from build123d import *

# Parameters (mm, degrees)
F0_W     = 67.3
F0_H     = 105.5
F1_DEPTH = 3
F2_W     = 56.2
F2_H     = 97.6
F3_DEPTH = 0.3
F4_W     = 48.5
F4_H     = 3
F5_DEPTH = 2


with BuildPart() as f1:
    # F0 (on Top) → F1 (new body)
    with BuildSketch(Plane.XY):
        with Locations((11.620628, 4.456163)):
            Rectangle(F0_W, F0_H)
    extrude(amount=F1_DEPTH)

    # F2 (on face) → F3 (cut)
    with BuildSketch(Plane.XY.offset(3)):
        with Locations((13.620628, 4.306163)):
            Rectangle(F2_W, F2_H)
    extrude(amount=-F3_DEPTH, mode=Mode.SUBTRACT)

    # F4 (on face) → F5 (join)
    with BuildSketch(Plane(origin=(-22.029372, 0, 0), x_dir=(0, -1, 0), z_dir=(-1, 0, 0))):
        with Locations((-14.056163, 1.5)):
            Rectangle(F4_W, F4_H)
    extrude(amount=F5_DEPTH)


solid = f1.part
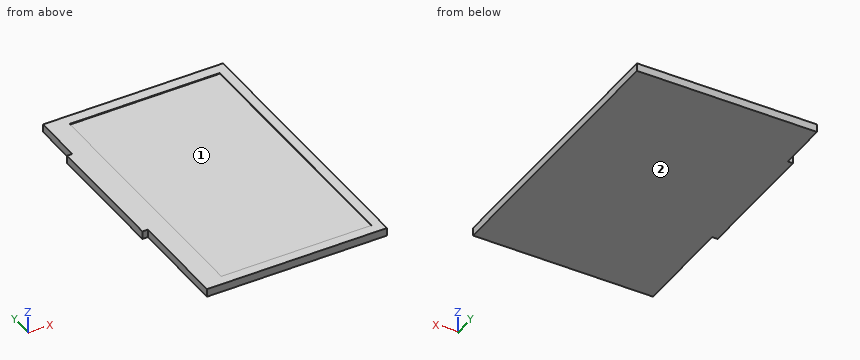
Verification items for the finished model (mm, model axes). Face numbers are marked on the shaded views. Coordinates: 2 decimals unless noted, no trailing zeros. Order: outer loops, then holes, each group sorted by start corner. A loop starts at its lowest first (then second) coordinate and runs counter-clockwise, first axis right, second up. Notation, with made-up numbers: (65, 76) -> (98, 76) arc R12 cw to (98, 85) -> close; hole circle Ø3 at (54.25, 83). An arc over 180 degrees is marked (long way). Use CSV: the item, a comma, the result in double quotes. Start each with the question number.
Q1. Section check B-B, the plane x = 11.5. Record the cut outline in (y, z), and give its area (3 significant figures).
Q2. Thickness scan on line 1 along Y through (x, z) = (31, 2.9); line 2 along Z through (x, y) = (29, 15.5); line 3 along X through (y, z) = (-12.5, 0.9). Record the ranges inside material, lowest first.
Q3. Depth check by flat-ended pin: P1, Ø1.5, axis at y = 47.5, z = 2, coming from the -X side; P2, Ø6, axis at x = 33.5, y = -2.5, coming from the +Z side; P3, Ø1.6, axis at x = -23, z = 1.5, coming from the +Y side; P4, Ø1.6, axis at x = -22.5, z = 1.5, coming from the -Y side. Enter the tip coordinate at first touch or a pass-through.
Q4. Section check A-A, the plane y = 22. Record the cut outline in (x, z).
Q5. Draft check along Y on the marked faces 1 and 2. Enter one of: +Y half, -Y half, draft (parallel to the pull), parting line (faces both ways), or undercut.
Returned:
1,outline,"(-48.29, 0) -> (57.21, 0) -> (57.21, 3) -> (53.11, 3) -> (53.11, 2.7) -> (-44.49, 2.7) -> (-44.49, 3) -> (-48.29, 3) -> close"
1,area,"287 mm^2"
2,line 1,"y = -48.29 to -44.49, 53.11 to 57.21"
2,line 2,"z = 0 to 2.7"
2,line 3,"x = -22.03 to 45.27"
3,P1,"stops at x = -22.03"
3,P2,"stops at z = 2.7"
3,P3,"stops at y = 38.31"
3,P4,"stops at y = -48.29"
4,outline,"(-24.03, 0) -> (45.27, 0) -> (45.27, 3) -> (41.72, 3) -> (41.72, 2.7) -> (-14.48, 2.7) -> (-14.48, 3) -> (-24.03, 3) -> close"
5,face 1,"undercut"
5,face 2,"draft"
